```python
from build123d import *

# Parameters (mm, degrees)
SKETCH1_W                        = 480
SKETCH1_H                        = 313
BASE_DEPTH                       = 4
SKETCH2_W                        = 20
SKETCH2_H                        = 5
TOP_TABS_DEFINITION_DEPTH        = 4
TOP_TABS_PATTERN_COUNT           = 5
TOP_TABS_PATTERN_PITCH           = 55
TOP_TABS_PATTERN_COL_COUNT       = 5
TOP_TABS_PATTERN_COL_PITCH       = 55
BOTTOM_TABS_COPY_1_SKETCH_W      = 20
BOTTOM_TABS_COPY_1_SKETCH_H      = 5
BOTTOM_TABS_COPY_1_DEPTH         = 4
BOTTOM_TABS_COPY_2_SKETCH_W      = 20
BOTTOM_TABS_COPY_2_SKETCH_H      = 5
BOTTOM_TABS_COPY_2_DEPTH         = 4
BOTTOM_TABS_COPY_3_SKETCH_W      = 20
BOTTOM_TABS_COPY_3_SKETCH_H      = 5
BOTTOM_TABS_COPY_3_DEPTH         = 4
BOTTOM_TABS_COPY_4_SKETCH_W      = 20
BOTTOM_TABS_COPY_4_SKETCH_H      = 5
BOTTOM_TABS_COPY_4_DEPTH         = 4
BOTTOM_TABS_COPY_5_SKETCH_W      = 20
BOTTOM_TABS_COPY_5_SKETCH_H      = 5
BOTTOM_TABS_COPY_5_DEPTH         = 4
BOTTOM_TABS_COPY_6_SKETCH_W      = 20
BOTTOM_TABS_COPY_6_SKETCH_H      = 5
BOTTOM_TABS_COPY_6_DEPTH         = 4
BOTTOM_TABS_COPY_7_SKETCH_W      = 20
BOTTOM_TABS_COPY_7_SKETCH_H      = 5
BOTTOM_TABS_COPY_7_DEPTH         = 4
BOTTOM_TABS_COPY_8_SKETCH_W      = 20
BOTTOM_TABS_COPY_8_SKETCH_H      = 5
BOTTOM_TABS_COPY_8_DEPTH         = 4
ELECTRONICS_MOUNTING_HOLES_1_5_D = 1.5
SKETCH7_W                        = 5
SKETCH7_H                        = 20
LEFT_TABS_DEFINITION_DEPTH       = 4
LEFT_TABS_PATTERN_COUNT          = 3
LEFT_TABS_PATTERN_PITCH          = 55
LEFT_TABS_PATTERN_COL_COUNT      = 3
LEFT_TABS_PATTERN_COL_PITCH      = 55
RIGHT_TABS_COPY_1_SKETCH_W       = 5
RIGHT_TABS_COPY_1_SKETCH_H       = 20
RIGHT_TABS_COPY_1_DEPTH          = 4
RIGHT_TABS_COPY_2_SKETCH_W       = 5
RIGHT_TABS_COPY_2_SKETCH_H       = 20
RIGHT_TABS_COPY_2_DEPTH          = 4
RIGHT_TABS_COPY_3_SKETCH_W       = 5
RIGHT_TABS_COPY_3_SKETCH_H       = 20
RIGHT_TABS_COPY_3_DEPTH          = 4
RIGHT_TABS_COPY_4_SKETCH_W       = 5
RIGHT_TABS_COPY_4_SKETCH_H       = 20
RIGHT_TABS_COPY_4_DEPTH          = 4
M6_CLEARANCE_HOLE1_D             = 5
TAP_DRILL_FOR_M3X0_5_TAP1_D      = 2.5


with BuildPart() as part:
    # Sketch1 → Base (new body)
    with BuildSketch(Plane(origin=(0, 0, 0), x_dir=(1, 0, 0), z_dir=(0, 1, 0))):
        Rectangle(SKETCH1_W, SKETCH1_H)
    extrude(amount=BASE_DEPTH)

    # Sketch2 → Top Tabs Definition (add)
    with BuildSketch(Plane(origin=(0, 4, 0), x_dir=(1, 0, 0), z_dir=(0, 1, 0))):
        with Locations((0, 159)):
            Rectangle(SKETCH2_W, SKETCH2_H)
    top_tabs_definition = extrude(amount=-TOP_TABS_DEFINITION_DEPTH)

    # Top Tabs Pattern: Top Tabs Definition ×5
    with Locations(*[(-i * TOP_TABS_PATTERN_PITCH, 0, 0) for i in range(1, TOP_TABS_PATTERN_COUNT)]):
        add(top_tabs_definition)

    # Top Tabs Pattern col: Top Tabs Definition ×5
    with Locations(*[(i * TOP_TABS_PATTERN_COL_PITCH, 0, 0) for i in range(1, TOP_TABS_PATTERN_COL_COUNT)]):
        add(top_tabs_definition)

    # Bottom Tabs: Top Tabs Definition across plane
    add(top_tabs_definition.mirror(Plane.XY))

    # Bottom Tabs copy 1 sketch → Bottom Tabs copy 1 (add)
    with BuildSketch(Plane(origin=(-55, 4, 0), x_dir=(1, 0, 0), z_dir=(0, 1, 0))):
        with Locations((0, -159)):
            Rectangle(BOTTOM_TABS_COPY_1_SKETCH_W, BOTTOM_TABS_COPY_1_SKETCH_H)
    extrude(amount=-BOTTOM_TABS_COPY_1_DEPTH)

    # Bottom Tabs copy 2 sketch → Bottom Tabs copy 2 (add)
    with BuildSketch(Plane(origin=(-110, 4, 0), x_dir=(1, 0, 0), z_dir=(0, 1, 0))):
        with Locations((0, -159)):
            Rectangle(BOTTOM_TABS_COPY_2_SKETCH_W, BOTTOM_TABS_COPY_2_SKETCH_H)
    extrude(amount=-BOTTOM_TABS_COPY_2_DEPTH)

    # Bottom Tabs copy 3 sketch → Bottom Tabs copy 3 (add)
    with BuildSketch(Plane(origin=(-165, 4, 0), x_dir=(1, 0, 0), z_dir=(0, 1, 0))):
        with Locations((0, -159)):
            Rectangle(BOTTOM_TABS_COPY_3_SKETCH_W, BOTTOM_TABS_COPY_3_SKETCH_H)
    extrude(amount=-BOTTOM_TABS_COPY_3_DEPTH)

    # Bottom Tabs copy 4 sketch → Bottom Tabs copy 4 (add)
    with BuildSketch(Plane(origin=(-220, 4, 0), x_dir=(1, 0, 0), z_dir=(0, 1, 0))):
        with Locations((0, -159)):
            Rectangle(BOTTOM_TABS_COPY_4_SKETCH_W, BOTTOM_TABS_COPY_4_SKETCH_H)
    extrude(amount=-BOTTOM_TABS_COPY_4_DEPTH)

    # Bottom Tabs copy 5 sketch → Bottom Tabs copy 5 (add)
    with BuildSketch(Plane(origin=(55, 4, 0), x_dir=(1, 0, 0), z_dir=(0, 1, 0))):
        with Locations((0, -159)):
            Rectangle(BOTTOM_TABS_COPY_5_SKETCH_W, BOTTOM_TABS_COPY_5_SKETCH_H)
    extrude(amount=-BOTTOM_TABS_COPY_5_DEPTH)

    # Bottom Tabs copy 6 sketch → Bottom Tabs copy 6 (add)
    with BuildSketch(Plane(origin=(110, 4, 0), x_dir=(1, 0, 0), z_dir=(0, 1, 0))):
        with Locations((0, -159)):
            Rectangle(BOTTOM_TABS_COPY_6_SKETCH_W, BOTTOM_TABS_COPY_6_SKETCH_H)
    extrude(amount=-BOTTOM_TABS_COPY_6_DEPTH)

    # Bottom Tabs copy 7 sketch → Bottom Tabs copy 7 (add)
    with BuildSketch(Plane(origin=(165, 4, 0), x_dir=(1, 0, 0), z_dir=(0, 1, 0))):
        with Locations((0, -159)):
            Rectangle(BOTTOM_TABS_COPY_7_SKETCH_W, BOTTOM_TABS_COPY_7_SKETCH_H)
    extrude(amount=-BOTTOM_TABS_COPY_7_DEPTH)

    # Bottom Tabs copy 8 sketch → Bottom Tabs copy 8 (add)
    with BuildSketch(Plane(origin=(220, 4, 0), x_dir=(1, 0, 0), z_dir=(0, 1, 0))):
        with Locations((0, -159)):
            Rectangle(BOTTOM_TABS_COPY_8_SKETCH_W, BOTTOM_TABS_COPY_8_SKETCH_H)
    extrude(amount=-BOTTOM_TABS_COPY_8_DEPTH)

    # Electronics Mounting Holes (1.5) (through all)
    with Locations(Plane(origin=(0, 4, 0), x_dir=(1, 0, 0), z_dir=(0, 1, 0))):
        with Locations((-142.5, 122.880889181), (-111.5, 122.880889181), (-111.5, 69.880889181), (-142.5, 69.880889181), (-161.5, 85.493748074), (-161.5, 146.493748074), (-222.5, 146.493748074), (-222.5, 85.493748074), (156.815, 133.05999982), (222.855, 136.23499982), (222.855, 87.97499982), (156.815, 91.14999982)):
            Hole(ELECTRONICS_MOUNTING_HOLES_1_5_D / 2)

    # Sketch7 → Left Tabs Definition (add)
    with BuildSketch(Plane(origin=(0, 4, 0), x_dir=(1, 0, 0), z_dir=(0, 1, 0))):
        with Locations((-242.5, 0)):
            Rectangle(SKETCH7_W, SKETCH7_H)
    left_tabs_definition = extrude(amount=-LEFT_TABS_DEFINITION_DEPTH)

    # Left Tabs Pattern: Left Tabs Definition ×3
    with Locations(*[(0, 0, -i * LEFT_TABS_PATTERN_PITCH) for i in range(1, LEFT_TABS_PATTERN_COUNT)]):
        add(left_tabs_definition)

    # Left Tabs Pattern col: Left Tabs Definition ×3
    with Locations(*[(0, 0, i * LEFT_TABS_PATTERN_COL_PITCH) for i in range(1, LEFT_TABS_PATTERN_COL_COUNT)]):
        add(left_tabs_definition)

    # Right Tabs: Left Tabs Definition across plane
    add(left_tabs_definition.mirror(Plane(origin=(0, 0, 0), x_dir=(0, 0, 1), z_dir=(1, 0, 0))))

    # Right Tabs copy 1 sketch → Right Tabs copy 1 (add)
    with BuildSketch(Plane(origin=(0, 4, -55), x_dir=(-1, 0, 0), z_dir=(0, 1, 0))):
        with Locations((-242.5, 0)):
            Rectangle(RIGHT_TABS_COPY_1_SKETCH_W, RIGHT_TABS_COPY_1_SKETCH_H)
    extrude(amount=-RIGHT_TABS_COPY_1_DEPTH)

    # Right Tabs copy 2 sketch → Right Tabs copy 2 (add)
    with BuildSketch(Plane(origin=(0, 4, -110), x_dir=(-1, 0, 0), z_dir=(0, 1, 0))):
        with Locations((-242.5, 0)):
            Rectangle(RIGHT_TABS_COPY_2_SKETCH_W, RIGHT_TABS_COPY_2_SKETCH_H)
    extrude(amount=-RIGHT_TABS_COPY_2_DEPTH)

    # Right Tabs copy 3 sketch → Right Tabs copy 3 (add)
    with BuildSketch(Plane(origin=(0, 4, 55), x_dir=(-1, 0, 0), z_dir=(0, 1, 0))):
        with Locations((-242.5, 0)):
            Rectangle(RIGHT_TABS_COPY_3_SKETCH_W, RIGHT_TABS_COPY_3_SKETCH_H)
    extrude(amount=-RIGHT_TABS_COPY_3_DEPTH)

    # Right Tabs copy 4 sketch → Right Tabs copy 4 (add)
    with BuildSketch(Plane(origin=(0, 4, 110), x_dir=(-1, 0, 0), z_dir=(0, 1, 0))):
        with Locations((-242.5, 0)):
            Rectangle(RIGHT_TABS_COPY_4_SKETCH_W, RIGHT_TABS_COPY_4_SKETCH_H)
    extrude(amount=-RIGHT_TABS_COPY_4_DEPTH)

    # M6 Clearance Hole1 (through all)
    with Locations(Plane(origin=(0, 4, 0), x_dir=(1, 0, 0), z_dir=(0, 1, 0))):
        with Locations((-147.5, 15.670311787), (-22.5, 15.670311787), (102.5, 15.670311787)):
            Hole(M6_CLEARANCE_HOLE1_D / 2)

    # Tap Drill for M3x0.5 Tap1 (through all)
    with Locations(Plane(origin=(0, 0, 0), x_dir=(-1, 0, 0), z_dir=(0, -1, 0))):
        with Locations((124, -117.946251926), (226, -97.946251926)):
            Hole(TAP_DRILL_FOR_M3X0_5_TAP1_D / 2)


solid = part.part
```
Check sheet for the modelled part. Datum: model origin and axes. Units: mm. Round coordinates to 2 decimals unless told otherwise and drop trailing zeros. Write each loop counter-clockwise with the first axis right and the second up, starting at its lowest first coordinate (ties: lowest second). Pieces come first, ordered by that corner, then holes. Notation, with made-up numbers: (-13.5, 80) -> (-8.5, 80) arc R9 ccw to (-8.5, 93) -> close; hole circle Ø11 at (-3.5, 78). An arc over 180 degrees is marked (long way). One line per question, with ' | ' between items. Start each with the question number.
1. Depth check by flat-ended pin: pin 1 (1 mm diameter, centred on y = 1, z = 121.5, fed in from +X); pin 2 (1.2 mm diameter, centred on x = -243, y = 2.5, fed in from -Z); pin 3 (2 mm diameter, centred on y = 1.5, z = -159, fed in from -X). Enter the tip coordinate at first touch or a pass-through.
2. Sectioned sample at C-C, the plane y = 2.65. Count the separate pieces of the cut face and the enclosed holes in it, then the cut area to 3 significant figures.
3. Scan lines: line 1 along Z through (x, y) = (-65.5, 1.3); line 2 along Z through (x, y) = (102.5, 1.7); line 3 along X through (y, z) = (2.2, -125). Record each from-to range of solid material in increasing order. Write a range as from..to.
4. Sectioned sample at A-A, the plane z = 24. Record the cut outline in (x, y), then the cut area to 3 significant figures.
5. Sectioned sample at B-B, the plane x = 28.5. Record the cut outline in (y, z), then the cut area to 3 significant figures.
Taken from the geometry:
1) pin 1: stops at x = 240 | pin 2: stops at z = -120 | pin 3: stops at x = -230
2) separate pieces: 1 | enclosed holes: 17 | area: 153,000 mm^2
3) line 1: z = -156.5..156.5 | line 2: z = -161.5..-18.17, -13.17..161.5 | line 3: x = -240..240
4) outline: (-240, 0) -> (240, 0) -> (240, 4) -> (-240, 4) -> close | area: 1,920 mm^2
5) outline: (0, -156.5) -> (4, -156.5) -> (4, 156.5) -> (0, 156.5) -> close | area: 1,250 mm^2
